```python
from build123d import *

# Parameters (mm, degrees)
SKETCH1_R           = 100
BOSS_EXTRUDE3_DEPTH = 140
BOSS_EXTRUDE3_TAPER = 31.3
SKETCH2_R           = 97.5
CUT_EXTRUDE1_DEPTH  = 140
CUT_EXTRUDE1_DRAFT  = -31.3
SKETCH4_R           = 15
SKETCH4_R_2         = 12.5
EXTRUDE_THIN1_DEPTH = 35


with BuildPart() as part:
    # Sketch1 → Boss-Extrude3 (new body)
    with BuildSketch(Plane(origin=(0, 0, 0), x_dir=(1, 0, 0), z_dir=(0, 1, 0))):
        Circle(SKETCH1_R)
    extrude(amount=BOSS_EXTRUDE3_DEPTH, taper=BOSS_EXTRUDE3_TAPER)


with BuildPart() as cut_extrude1_tool:
    # Sketch2 → Cut-Extrude1 (with draft: the straight prism first)
    with BuildSketch(Plane.XZ):
        Circle(SKETCH2_R)
    extrude(amount=-CUT_EXTRUDE1_DEPTH)
    # Cut-Extrude1: the draft: its side faces are tilted about the plane it starts from
    cut_extrude1_sides = [cut_extrude1_tool.faces().sort_by_distance(p)[0] for p in [
        (-97.5, 70, 0),
    ]]
    draft(cut_extrude1_sides, Plane.XZ, CUT_EXTRUDE1_DRAFT)


with BuildPart() as part_1:
    add(part.part)

    # Cut-Extrude1: cut by cut_extrude1_tool
    add(cut_extrude1_tool.part, mode=Mode.SUBTRACT)

    # Sketch4 → Extrude-Thin1 (add)
    with BuildSketch(Plane(origin=(0, 140, 0), x_dir=(1, 0, 0), z_dir=(0, 1, 0))):
        Circle(SKETCH4_R)
        Circle(SKETCH4_R_2, mode=Mode.SUBTRACT)
    extrude(amount=EXTRUDE_THIN1_DEPTH)


solid = part_1.part
```
Verification items for the finished model (mm, model axes). A direction names the side the tool comes from. Give positions to 0.01 mm unless a question says otherwise; leave off trailing zeros. Order: outer loops, then holes, each group sorted by start corner. A loop starts at its lowest first (then second) coordinate and runs counter-clockwise, first axis right, second up. Notation, with made-up numbers: (40, -1) - (57, -1) arc R25 ccw to (57, 17) - close; hole circle Ø9 at (26, 42.25). An arc over 180 degrees is marked (long way). Answer as CSV lines item,"result". Start each with the question number.
Item 1: Access from +Z, -Z, +X, -X, +Y, -Y to the whole of each face (thin tool, end or side, straight path). Record for faces 4 (the face through (-14.985, 157.255, -0.66)), 5 (the face through (-3.4, 175, -12.3)).
Item 2: Section check B-B, the plane x = 0. Record the boundary of the cut face in (y, z).
Item 3: Material ranges on L1, parallel to Z at x = 0, y = 148.5; L2, parallel to Z at x = -9, y = 90.5, recorded low to high.
Item 4: Mould release check, pull along X, two halves, no side actions. Record for faces 1 (the face through (96, 0, 22)), 2 (the face through (11.923, 157.255, -3.755)), 3 (the face through (-4.937, 102.091, -37.605)): released by +X, released by -X, zero draft, split by the parting line, or undercut.
Item 5: Gauge pin test, flat ends, axial feed: pin 1 (2 mm diameter, centred on y = 18.5, z = 61, fed in from +X); pin 2 (10 mm diameter, centred on x = -12.5, z = -69, fed in from +Y); pin 3 (20 mm diameter, centred on x = 0, z = 0, fed in from +Y); pin 4 (15 mm diameter, centred on x = -5, z = -4.5, fed in from -Y). Record the tip position at first contact, or that the pin passes through.
Item 6: Section check A-A, the plane y = 154. Record the boundary of the cut face in (x, z), plus the area to 3 significant figures.
Item 7: Section check C-C, the plane y = 120. Record the boundary of the cut face in (x, z).
Filled in:
1,face 4,"+Y"
1,face 5,"+Z, -Z, +X, -X, +Y"
2,outline,"(0, -100) - (140, -14.88) - (140, -15) - (175, -15) - (175, -12.5) - (140, -12.5) - (140, -12.38) - (0, -97.5) - close; (0, 97.5) - (140, 12.38) - (140, 12.5) - (175, 12.5) - (175, 15) - (140, 15) - (140, 14.88) - (0, 100) - close"
3,L1,"-15 to -12.5, 12.5 to 15"
3,L2,"-44.07 to -41.51, 41.51 to 44.07"
4,face 1,"zero draft"
4,face 2,"undercut"
4,face 3,"split by the parting line"
5,pin 1,"x = 65.71"
5,pin 2,"y = 57.36"
5,pin 3,"through"
5,pin 4,"y = 136.96"
6,outline,"circle Ø30 at (0, 0); hole circle Ø25 at (0, 0)"
6,area,"216 mm^2"
7,outline,"circle Ø54.08 at (0, 0); hole circle Ø49.08 at (0, 0)"
